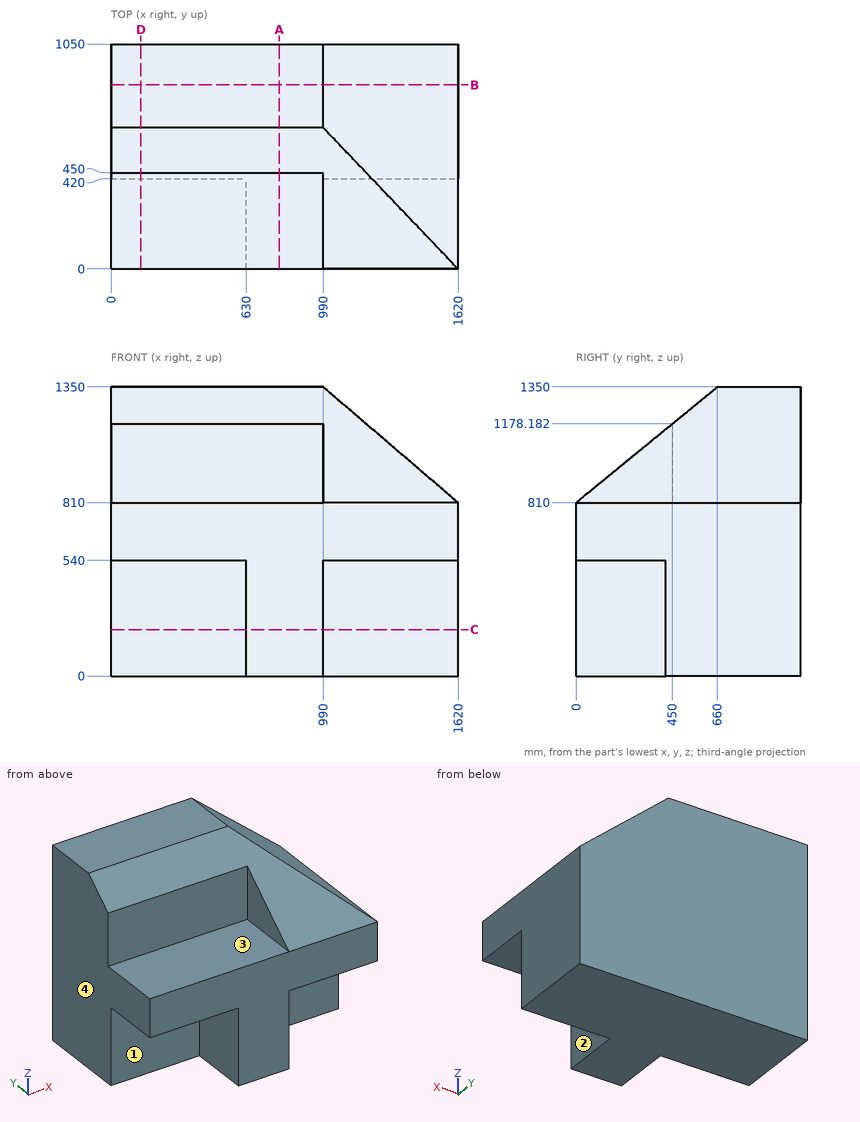
Design review of the part shown in the three views and the two pictorial views. Dimensions are in mm from the part's minimum x, y and z. A direction names the side the tool comes from. Coordinates: 2 decimals unless noted, no trailing zeros. Order: outer loops, then holes, each group sorted by start corner. A loop starts at its lowest first (then second) coordinate and runs counter-clockwise, first axis right, second up.
Item 1: Take a section at A-A, the plane x = 785.5. Write out the cut boundary in (y, z), then the cut area to 3 significant figures.
Item 2: Take a section at B-B, the plane y = 859.5. Write out the cut boundary in (x, z), then the cut area to 3 significant figures.
Item 3: For line 1 (Y direction, x = 549, z = 202); line 2 (Z direction, x = 249, y = 179); line 3 (X direction, y = 259, z = 278), list the stretches that pass through material, from the lowest coordinate up.
Item 4: For pin 1 Ø2 at (x, z) = (1345, 237) entering from -Y, flat-tipped, find the tip position at first contact; note if it passes through.
Item 5: Take a section at D-D, the plane x = 139. Write out the cut boundary in (y, z), then the cut area to 3 significant figures.
Item 6: For the marked faces 1, 2, 3 and 4, list the 3-axis set-ups (+Z, -Z, +X, -X, +Y, -Y) from which the entire face can be reached by the end or side of a thin tool; tool diameter is ignored.
Item 7: Take a section at C-C, the plane z = 217. Write out the cut boundary in (x, y).
The answers:
1. outline: (0, 0) - (1050, 0) - (1050, 1350) - (660, 1350) - (450, 1178.18) - (450, 810) - (0, 810) - close
1. area: 1,160,000 mm2
2. outline: (0, 0) - (1620, 0) - (1620, 810) - (990, 1350) - (0, 1350) - close
2. area: 2,020,000 mm2
3. line 1: y = 420 to 1050
3. line 2: z = 540 to 810
3. line 3: x = 630 to 990
4. pin 1: stops at y = 420
5. outline: (0, 540) - (420, 540) - (420, 0) - (1050, 0) - (1050, 1350) - (660, 1350) - (450, 1178.18) - (450, 810) - (0, 810) - close
5. area: 930,000 mm2
6. face 1: -Z, -X, -Y
6. face 2: -Z, +X, -Y
6. face 3: +Z, -X, -Y
6. face 4: +Z, -Z, -X, +Y, -Y
7. outline: (0, 420) - (630, 420) - (630, 0) - (990, 0) - (990, 420) - (1620, 420) - (1620, 1050) - (0, 1050) - close
